Here's how the part is built. I have some questions about the finished solid (model axes, mm). A direction names the side the tool comes from. Round coordinates to 2 decimals unless told otherwise and drop trailing zeros. Loops run counter-clockwise (first coordinate to the right, second up) from the corner with the lowest first, then second, coordinate; pieces in that order, holes last. Notation, with made-up numbers: M 7,54.5 L 57,54.5 A19 ccw 57,73.5 Z; hole C 43,77.5 d11. An arc over 180 degrees is marked long. Write item = value, one per line. Start each with the question number.
from build123d import *

# Parameters (mm, degrees)
IZIM1_W                     = 260
IZIM1_H                     = 115
IZIM1_W_2                   = 240
IZIM1_H_2                   = 90
Y_KSEKLIK_EKSTR_ZYON1_DEPTH = 10
Y_KSEKLIK_EKSTR_ZYON2_START = -12.5
Y_KSEKLIK_EKSTR_ZYON2_DEPTH = 12.5
IZIM3_W                     = 10
IZIM3_H                     = 12.5
Y_KSEKLIK_EKSTR_ZYON3_DEPTH = 50
IZIM4_R                     = 2.5
Y_KSEKLIK_EKSTR_ZYON4_DEPTH = 15
IZIM5_R                     = 0.75
KES_EKSTR_ZYON1_DEPTH       = 15
PAH1_SIZE                   = 0.75
IZIM6_R                     = 2.5
Y_KSEKLIK_EKSTR_ZYON5_DEPTH = 15
IZIM7_R                     = 0.75
KES_EKSTR_ZYON2_DEPTH       = 15
PAH2_SIZE                   = 0.75
PAH3_SIZE                   = 0.75
IZIM8_R                     = 2.5
KES_EKSTR_ZYON3_DEPTH       = 15
IZIM9_R                     = 3.5
KES_EKSTR_ZYON4_DEPTH       = 15


with BuildPart() as part:
    # Çizim1 → Yükseklik-Ekstrüzyon1 (new body)
    with BuildSketch(Plane.XY):
        with Locations((130, 57.5)):
            Rectangle(IZIM1_W, IZIM1_H)
        with Locations((130, 57.5)):
            Rectangle(IZIM1_W_2, IZIM1_H_2, mode=Mode.SUBTRACT)
    extrude(amount=Y_KSEKLIK_EKSTR_ZYON1_DEPTH)

    # Çizim2 → Yükseklik-Ekstrüzyon2 (add)
    with BuildSketch(Plane(origin=(0, 115, 0), x_dir=(1, 0, 0), z_dir=(0, 1, 0)).offset(Y_KSEKLIK_EKSTR_ZYON2_START)):
        Polygon((260, -10), (260, -50), (50, -50), (50, -10), (60, -10), (60, -40), (250, -40), (250, -10), align=None)
    extrude(amount=Y_KSEKLIK_EKSTR_ZYON2_DEPTH)

    # Çizim3 → Yükseklik-Ekstrüzyon3 (add)
    with BuildSketch(Plane.XY.offset(50)):
        with Locations((255, 108.75)):
            Rectangle(IZIM3_W, IZIM3_H)
        with Locations((135, 108.75)):
            Rectangle(IZIM3_W, IZIM3_H)
    extrude(amount=Y_KSEKLIK_EKSTR_ZYON3_DEPTH)

    # Çizim4 → Yükseklik-Ekstrüzyon4 (add)
    with BuildSketch(Plane(origin=(260, 0, 0), x_dir=(0, 0, -1), z_dir=(1, 0, 0))):
        with Locations(Location((-90, 108.75, 0), (0, 0, 180))):
            Circle(IZIM4_R)
    y_kseklik_ekstr_zyon4 = extrude(amount=Y_KSEKLIK_EKSTR_ZYON4_DEPTH)

    # Çizim5 → Kes-Ekstrüzyon1 (cut)
    with BuildSketch(Plane(origin=(0, 115, 0), x_dir=(1, 0, 0), z_dir=(0, 1, 0))):
        with Locations(Location((271, -90, 0), (0, 0, 270))):
            Circle(IZIM5_R)
    kes_ekstr_zyon1 = extrude(amount=-KES_EKSTR_ZYON1_DEPTH, mode=Mode.SUBTRACT)

    # Aynalama1: Yükseklik-Ekstrüzyon4, Kes-Ekstrüzyon1 across plane
    add(y_kseklik_ekstr_zyon4.mirror(Plane(origin=(195, 0, 0), x_dir=(0, 0, 1), z_dir=(1, 0, 0))))
    add(kes_ekstr_zyon1.mirror(Plane(origin=(195, 0, 0), x_dir=(0, 0, 1), z_dir=(1, 0, 0))), mode=Mode.SUBTRACT)

    # Pah1
    pah1_edges = [part.edges().sort_by_distance(p)[0] for p in [
        (275, 108.75, 87.5),
        (115, 108.75, 87.5),
    ]]
    chamfer(pah1_edges, length=PAH1_SIZE)

    # Çizim6 → Yükseklik-Ekstrüzyon5 (add)
    with BuildSketch(Plane(origin=(260, 0, 0), x_dir=(0, 0, -1), z_dir=(1, 0, 0))):
        with Locations(Location((-5, 5, 0), (0, 0, 180))):
            Circle(IZIM6_R)
    y_kseklik_ekstr_zyon5 = extrude(amount=Y_KSEKLIK_EKSTR_ZYON5_DEPTH)

    # Çizim7 → Kes-Ekstrüzyon2 (cut)
    with BuildSketch(Plane.XZ):
        with Locations(Location((273, 5, 0), (0, 0, 270))):
            Circle(IZIM7_R)
    kes_ekstr_zyon2 = extrude(amount=-KES_EKSTR_ZYON2_DEPTH, mode=Mode.SUBTRACT)

    # Pah2
    pah2_edges = [part.edges().sort_by_distance(p)[0] for p in [
        (275, 5, 2.5),
    ]]
    chamfer(pah2_edges, length=PAH2_SIZE)

    # Aynalama5: Yükseklik-Ekstrüzyon5, Kes-Ekstrüzyon2 across plane
    add(y_kseklik_ekstr_zyon5.mirror(Plane(origin=(130, 0, 0), x_dir=(0, 0, 1), z_dir=(1, 0, 0))))
    add(kes_ekstr_zyon2.mirror(Plane(origin=(130, 0, 0), x_dir=(0, 0, 1), z_dir=(1, 0, 0))), mode=Mode.SUBTRACT)

    # Pah3
    pah3_edges = [part.edges().sort_by_distance(p)[0] for p in [
        (-15, 5, 2.5),
    ]]
    chamfer(pah3_edges, length=PAH3_SIZE)

    # Çizim8 → Kes-Ekstrüzyon3 (cut)
    with BuildSketch(Plane(origin=(0, 115, 0), x_dir=(1, 0, 0), z_dir=(0, 1, 0))):
        with Locations(Location((210, -5, 0), (0, 0, 270))):
            Circle(IZIM8_R)
        with Locations(Location((180, -5, 0), (0, 0, 270))):
            Circle(IZIM8_R)
        with Locations(Location((105, -5, 0), (0, 0, 270))):
            Circle(IZIM8_R)
        with Locations(Location((75, -5, 0), (0, 0, 270))):
            Circle(IZIM8_R)
        with Locations(Location((75, -44.884971075, 0), (0, 0, 270))):
            Circle(IZIM8_R)
        with Locations(Location((105, -44.884971075, 0), (0, 0, 270))):
            Circle(IZIM8_R)
        with Locations(Location((180, -44.884971075, 0), (0, 0, 270))):
            Circle(IZIM8_R)
        with Locations(Location((210, -44.884971075, 0), (0, 0, 270))):
            Circle(IZIM8_R)
    extrude(amount=-KES_EKSTR_ZYON3_DEPTH, mode=Mode.SUBTRACT)

    # Çizim9 → Kes-Ekstrüzyon4 (cut)
    with BuildSketch(Plane.XY.offset(10)):
        with Locations((155, 107.5)):
            Circle(IZIM9_R)
        with Locations((25, 107.5)):
            Circle(IZIM9_R)
    extrude(amount=-KES_EKSTR_ZYON4_DEPTH, mode=Mode.SUBTRACT)


solid = part.part
Item 1: Will these pins go through, and if not, where does the flat tip stop? pin 1 Ø14 at (y, z) = (108, 29) entering from +X; pin 2 Ø14 at (x, y) = (119, 107.5) entering from +Z; pin 3 Ø6 at (x, z) = (105, 5) entering from -Y; pin 4 Ø1.4 at (x, z) = (271, 90) entering from -Y.
Item 2: Please list where these lines run through material, in increasing order: line 1 (Y direction, x = 155, z = 4); line 2 (Z direction, x = 111.5, y = 109); line 3 (X direction, y = 110, z = 26). Write a range as [from, to].
Item 3: I want a section at C-C, the plane y = 63. List the corners of the cut face in (x, z) for me, then the cut area to 3 significant figures.
Item 4: For faces 4 (the flat face through (196, 109, 50)), 5 (the cylindrical face through (107.48, 108.84, 4.67)), 6 (the cylindrical face through (122.97, 106.27, 89.67)), 7 (the flat face through (50, 109, 30)), 8 (the flat face through (250, 109, 25)), which set-ups out of +Z, -Z, +X, -X, +Y, -Y let a thin tool reach every point of the face, with its end or its side?
Item 5: We'd pull the mould along X, two halves only. Please class faces 1 (the cylindrical face through (212.48, 108.84, 4.67)), 2 (the flat face through (260, 79, 9)), 3 (the flat face through (120, 11, 10)): released by +X, released by -X, zero draft, split by the parting line, or undercut.
Item 6: I want a section at A-A, the plane z = 71. List the corners of the cut face in (x, y) for me, then the cut area to 3 significant figures.
Item 7: I want a section at B-B, the plane x = 84. List the corners of the cut face in (y, z) for me.
Item 8: I want a section at D-D, the plane x = 123. List the corners of the cut face in (y, z) for me, then the cut area to 3 significant figures.
Worked out:
q1.pin_1 = 260
q1.pin_2 = 92.5
q1.pin_3 = 0
q1.pin_4 = through
q2.line_1 = [0, 12.5], [102.5, 104], [111, 115]
q2.line_2 = [0, 10], [40, 50]
q2.line_3 = [50, 60], [250, 260]
q3.outline = M 0,0 L 10,0 L 10,10 L 0,10 Z; M 250,0 L 260,0 L 260,10 L 250,10 Z
q3.area = 200 mm2
q4.face_4 = +Z, +Y, -Y
q4.face_5 = +Y
q4.face_6 = -X
q4.face_7 = +Z, -X, +Y, -Y
q4.face_8 = +Y, -Y
q5.face_1 = undercut
q5.face_2 = released by +X
q5.face_3 = zero draft
q6.outline = M 130,102.5 L 140,102.5 L 140,115 L 130,115 Z; M 250,102.5 L 260,102.5 L 260,115 L 250,115 Z
q6.area = 250 mm2
q7.outline = M 0,0 L 12.5,0 L 12.5,10 L 0,10 Z; M 102.5,0 L 115,0 L 115,10 L 102.5,10 Z; M 102.5,40 L 115,40 L 115,50 L 102.5,50 Z
q8.outline = M 0,0 L 12.5,0 L 12.5,10 L 0,10 Z; M 102.5,0 L 115,0 L 115,10 L 102.5,10 Z; M 102.5,40 L 115,40 L 115,50 L 102.5,50 Z; C 108.75,90 d5
q8.area = 395 mm2
